Here's the drawing with two shaded views (mm, measured from the low corner). I have some questions. Round coordinates to 2 decimals unless told otherwise and drop trailing zeros. Order: outer loops, then holes, each group sorted by start corner. A loop starts at its lowest first (then second) coordinate and runs counter-clockwise, first axis right, second up. Notation, with made-up numbers: (86, -24.75) - (95, -24.75) arc R20 ccw to (95, 8.25) - close; hole circle Ø7 at (58, -19). An arc over 180 degrees is marked (long way). Return JSON: item names as keys, results as strings. Group by question number.
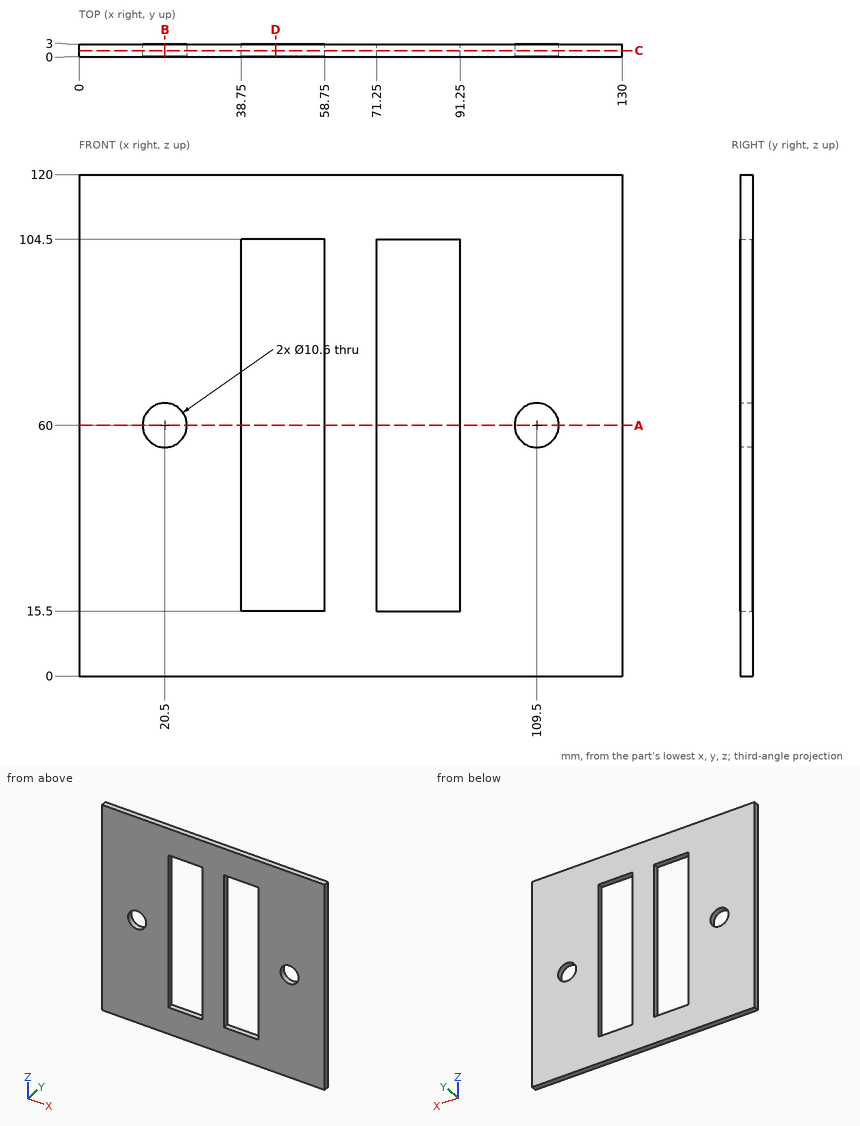
1) I want a section at B-B, the plane x = 20.5. List the corners of the cut face in (y, z) for me, plus the area to 3 significant figures.
2) I want a section at D-D, the plane x = 47. List the corners of the cut face in (y, z) for me, plus the area to 3 significant figures.
3) I want a section at A-A, the plane z = 60. List the corners of the cut face in (x, y) for me.
4) Will these pins go through, and if not, where does the flat tip stop? pin 1 (0.9 mm diameter, centred on x = 49.5, y = 1.5, fed in from -Z); pin 2 (8.5 mm diameter, centred on x = 109.5, z = 60, fed in from +Y).
5) I want a section at C-C, the plane y = 1.4. List the corners of the cut face in (x, z) for me.
6) If I drill on line 1 along X through (y, z) = (2, 78.5); line 2 along Z through (x, y) = (109.5, 1.3); line 3 along Z through (x, y) = (87.5, 2.8), over which ranges is the centre line in solid material (lowest first)? Write a range as from..to.
Outcome:
{
 "1": {"outline": "(0, 0) - (3, 0) - (3, 54.7) - (0, 54.7) - close; (0, 65.3) - (3, 65.3) - (3, 120) - (0, 120) - close", "area": "328 mm^2"},
 "2": {"outline": "(0, 0) - (3, 0) - (3, 15.5) - (0, 15.5) - close; (0, 104.5) - (3, 104.5) - (3, 120) - (0, 120) - close", "area": "93.0 mm^2"},
 "3": {"outline": "(0, 0) - (15.2, 0) - (15.2, 3) - (0, 3) - close; (25.8, 0) - (38.75, 0) - (38.75, 3) - (25.8, 3) - close; (58.75, 0) - (71.25, 0) - (71.25, 3) - (58.75, 3) - close; (91.25, 0) - (104.2, 0) - (104.2, 3) - (91.25, 3) - close; (114.8, 0) - (130, 0) - (130, 3) - (114.8, 3) - close"},
 "4": {"pin 1": "z = 0", "pin 2": "through"},
 "5": {"outline": "(0, 0) - (130, 0) - (130, 120) - (0, 120) - close; hole circle Ø10.6 at (20.5, 60); hole (38.75, 15.5) - (58.75, 15.5) - (58.75, 104.5) - (38.75, 104.5) - close; hole (71.25, 15.5) - (91.25, 15.5) - (91.25, 104.5) - (71.25, 104.5) - close; hole circle Ø10.6 at (109.5, 60)"},
 "6": {"line 1": "0..38.75, 58.75..71.25, 91.25..130", "line 2": "0..54.7, 65.3..120", "line 3": "0..15.5, 104.5..120"}
}
